Here's how the part is built. I have some questions about the finished solid (model axes, mm). Give positions to 0.01 mm unless a question says otherwise; leave off trailing zeros. Loops run counter-clockwise (first coordinate to the right, second up) from the corner with the lowest first, then second, coordinate; pieces in that order, holes last. Notation, with made-up numbers: M 29.5,71 L 69.5,71 A21 ccw 69.5,95 Z; hole C 54,54 d7. An arc over 180 degrees is marked long. Write item = value, one per line. Start each with the question number.
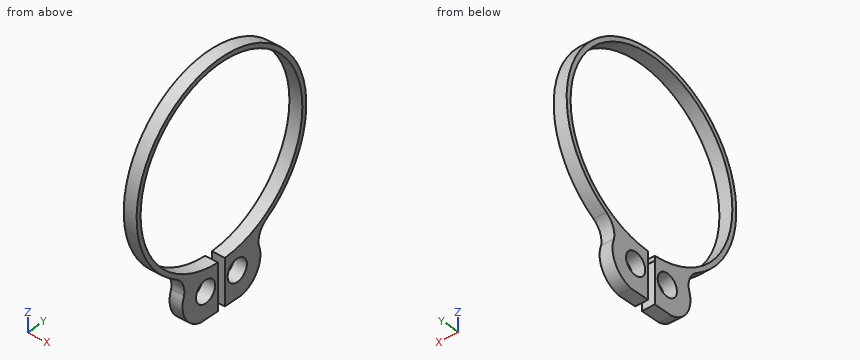
```python
from build123d import *

# Parameters (mm, degrees)
F0_R     = 0.85
F1_DEPTH = 1


with BuildPart() as f1:
    # F0 (on Right) → F1 (new body)
    with BuildSketch(Plane.YZ):
        with BuildLine():
            ThreePointArc((-0.3, -7.143704), (0, 7.15), (0.3, -7.143704))
            Line((0.3, -7.143704), (0.3, -10.65))
            Line((0.3, -10.65), (1.8, -10.65))
            ThreePointArc((1.8, -10.65), (3.195251, -9.624672), (3.304501, -7.896642))
            ThreePointArc((3.304501, -7.896642), (3.40666, -7.021654), (3.982704, -6.355161))
            ThreePointArc((3.982704, -6.355161), (0, 7.5), (-3.982704, -6.355161))
            ThreePointArc((-3.982704, -6.355161), (-3.40666, -7.021654), (-3.304501, -7.896642))
            ThreePointArc((-3.304501, -7.896642), (-3.195251, -9.624672), (-1.8, -10.65))
            Line((-1.8, -10.65), (-0.3, -10.65))
            Line((-0.3, -10.65), (-0.3, -7.505624))
            Line((-0.3, -7.505624), (-0.3, -7.493998))
            Line((-0.3, -7.493998), (-0.3, -7.143704))
        make_face()
        with Locations((-1.4, -8.643704)):
            Circle(F0_R, mode=Mode.SUBTRACT)
        with Locations((1.4, -8.643704)):
            Circle(F0_R, mode=Mode.SUBTRACT)
        with BuildLine():
            ThreePointArc((-0.292364, -7.494299), (-0.296182, -7.494149), (-0.3, -7.493998))
            Line((-0.3, -7.493998), (-0.3, -7.505624))
            ThreePointArc((-0.3, -7.505624), (-0.296191, -7.499955), (-0.292364, -7.494299))
        make_face()
    extrude(amount=-F1_DEPTH)


solid = f1.part
```
Q1. If we section it at C-C, the plane z = -8.25: List the corners of the cut face in (x, y) for me, then the cut area to 3 significant figures.
Q2. Will these pins go through, and if not, where does the flat tip stop? pin 1 (0.5 mm diameter, centred on x = -0.5, z = -8.5, fed in from +Y); pin 2 (1.5 mm diameter, centred on y = -1.4, z = -8.64, fed in from -X); pin 3 (0.5 mm diameter, centred on x = -0.5, z = -8.5, fed in from -Y).
Q3. If I drill on line 1 along Z through (x, y) = (-0.2, -1.4); line 2 along Y through (x, z) = (-0.75, 0); line 3 along Z through (x, y) = (-0.8, 3), over which ranges is the centre line in solid material (lowest first)?
Q4. If we section it at B-B, the plane y = 4.75: List the corners of the cut face in (x, z) for me.
Q5. If we section it at A-A, the plane z = 0: List the corners of the cut face in (x, y) for me.
Q6. If we section it at D-D, the plane y = 1.4: List the corners of the cut face in (x, z) for me.
Resolved:
q1.outline = M -1,-3.41 L 0,-3.41 L 0,-2.15 L -1,-2.15 Z; M -1,-0.65 L 0,-0.65 L 0,-0.3 L -1,-0.3 Z; M -1,0.3 L 0,0.3 L 0,0.65 L -1,0.65 Z; M -1,2.15 L 0,2.15 L 0,3.41 L -1,3.41 Z
q1.area = 3.20 mm²
q2.pin_1 = 3.45
q2.pin_2 = through
q2.pin_3 = -3.45
q3.line_1 = -10.65 to -9.49, -7.79 to -7.01, 7.01 to 7.37
q3.line_2 = -7.5 to -7.15, 7.15 to 7.5
q3.line_3 = -9.92 to -6.49, 6.49 to 6.87
q4.outline = M -1,-5.8 L 0,-5.8 L 0,-5.34 L -1,-5.34 Z; M -1,5.34 L 0,5.34 L 0,5.8 L -1,5.8 Z
q5.outline = M -1,-7.5 L 0,-7.5 L 0,-7.15 L -1,-7.15 Z; M -1,7.15 L 0,7.15 L 0,7.5 L -1,7.5 Z
q6.outline = M -1,-10.65 L 0,-10.65 L 0,-9.49 L -1,-9.49 Z; M -1,-7.79 L 0,-7.79 L 0,-7.01 L -1,-7.01 Z; M -1,7.01 L 0,7.01 L 0,7.37 L -1,7.37 Z
